from build123d import *

# Parameters (mm, degrees)
SKETCH1_R           = 14.3002
BOSS_EXTRUDE1_DEPTH = 69.85
SKETCH2_W           = 25.4
SKETCH2_H           = 44.45
CUT_EXTRUDE1_DEPTH  = 44.45
FILLET1_R           = 3.175
SKETCH3_R           = 2.921
CUT_EXTRUDE2_DEPTH  = 107.823534499
SKETCH4_R           = 2.921
CUT_EXTRUDE3_DEPTH  = 107.823534499
SKETCH5_R           = 4.445
CUT_EXTRUDE4_DEPTH  = 6.35
CUT_EXTRUDE5_DEPTH  = 7.62


with BuildPart() as part:
    # Sketch1 → Boss-Extrude1 (new body)
    with BuildSketch(Plane(origin=(0, 0, 0), x_dir=(0, 0, -1), z_dir=(1, 0, 0))):
        with BuildLine():
            Line((0, 0), (57.15, 0))
            Line((57.15, 0), (57.15, 38.1))
            ThreePointArc((57.15, 38.1), (51.570384182, 51.570384182), (38.1, 57.15))
            Line((38.1, 57.15), (0, 57.15))
            Line((0, 57.15), (0, 0))
        make_face()
        with Locations((31.75, 31.75)):
            Circle(SKETCH1_R, mode=Mode.SUBTRACT)
    extrude(amount=BOSS_EXTRUDE1_DEPTH)

    # Sketch2 → Cut-Extrude1 (cut)
    with BuildSketch(Plane(origin=(0, 57.15, 0), x_dir=(1, 0, 0), z_dir=(0, 1, 0))):
        with Locations((12.7, 34.925)):
            Rectangle(SKETCH2_W, SKETCH2_H)
        with Locations((57.15, 34.925)):
            Rectangle(SKETCH2_W, SKETCH2_H)
    extrude(amount=-CUT_EXTRUDE1_DEPTH, mode=Mode.SUBTRACT)

    # Fillet1
    fillet1_edges = [part.edges().sort_by_distance(p)[0] for p in [
        (69.85, 6.35, -57.15),
        (0, 57.15, -6.35),
        (69.85, 57.15, -6.35),
        (0, 12.7, -34.925),
        (0, 34.925, -12.7),
        (25.4, 25.4, -57.15),
        (25.4, 51.570384182, -51.570384182),
        (25.4, 12.7, -34.925),
        (12.7, 12.7, -57.15),
        (12.7, 12.7, -12.7),
        (25.4, 34.925, -12.7),
        (25.4, 57.15, -25.4),
        (12.7, 57.15, -12.7),
        (44.45, 51.570384182, -51.570384182),
        (44.45, 12.7, -34.925),
        (44.45, 34.925, -12.7),
        (69.85, 12.7, -34.925),
        (57.15, 12.7, -12.7),
        (69.85, 34.925, -12.7),
        (57.15, 12.7, -57.15),
        (44.45, 25.4, -57.15),
        (44.45, 57.15, -25.4),
        (57.15, 57.15, -12.7),
        (0, 6.35, -57.15),
        (34.925, 57.15, 0),
    ]]
    fillet(fillet1_edges, radius=FILLET1_R)

    # Sketch3 → Cut-Extrude2 (cut, through all)
    with BuildSketch(Plane.XY):
        with Locations((9.525, 25.4)):
            Circle(SKETCH3_R)
        with Locations((60.325, 25.4)):
            Circle(SKETCH3_R)
    extrude(amount=-CUT_EXTRUDE2_DEPTH, mode=Mode.SUBTRACT)

    # Sketch4 → Cut-Extrude3 (cut, through all)
    with BuildSketch(Plane.XZ):
        with Locations(Location((57.15, -25.4, 0), (0, 0, 270))):
            Circle(SKETCH4_R)
        with Locations(Location((57.15, -44.45, 0), (0, 0, 270))):
            Circle(SKETCH4_R)
        with Locations(Location((12.7, -25.4, 0), (0, 0, 270))):
            Circle(SKETCH4_R)
        with Locations(Location((12.7, -44.45, 0), (0, 0, 270))):
            Circle(SKETCH4_R)
    extrude(amount=-CUT_EXTRUDE3_DEPTH, mode=Mode.SUBTRACT)

    # Sketch5 → Cut-Extrude4 (cut)
    with BuildSketch(Plane(origin=(0, 12.7, 0), x_dir=(1, 0, 0), z_dir=(0, 1, 0))):
        with Locations(Location((12.7, 25.4, 0), (0, 0, 270))):
            Circle(SKETCH5_R)
        with Locations(Location((12.7, 44.45, 0), (0, 0, 270))):
            Circle(SKETCH5_R)
        with Locations(Location((57.15, 44.45, 0), (0, 0, 270))):
            Circle(SKETCH5_R)
        with Locations(Location((57.15, 25.4, 0), (0, 0, 270))):
            Circle(SKETCH5_R)
    extrude(amount=-CUT_EXTRUDE4_DEPTH, mode=Mode.SUBTRACT)

    # Sketch6 → Cut-Extrude5 (cut)
    with BuildSketch(Plane(origin=(0, 0, -12.7), x_dir=(-1, 0, 0), z_dir=(0, 0, -1))):
        Polygon((-57.392060633, 30.48), (-63.257939367, 30.48), (-66.190878735, 25.4), (-63.257939367, 20.32), (-57.392060633, 20.32), (-54.459121265, 25.4), align=None)
        Polygon((-6.592060633, 30.48), (-12.457939367, 30.48), (-15.390878735, 25.4), (-12.457939367, 20.32), (-6.592060633, 20.32), (-3.659121265, 25.4), align=None)
    extrude(amount=-CUT_EXTRUDE5_DEPTH, mode=Mode.SUBTRACT)


solid = part.part
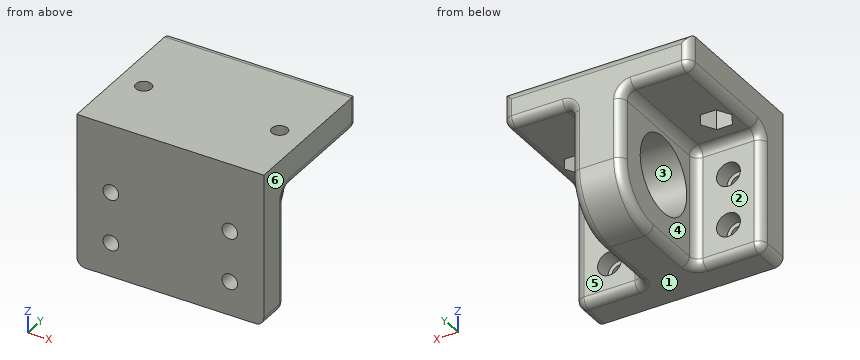
The listing builds one solid part. Answer for the finished solid, in the listing's coordinates (mm). Face numbers are marked on the shaded views. A direction names the side the tool comes from. Coordinates: 2 decimals unless noted, no trailing zeros. Write each loop counter-clockwise with the first axis right and the second up, starting at its lowest first coordinate (ties: lowest second). Pieces come first, ordered by that corner, then holes. Notation, with made-up numbers: M 46.5,36 L 99.5,36 A20 ccw 99.5,40 Z; hole C -24.75,6.25 d9. An arc over 180 degrees is marked long. Put each result on its own line as item: value. Start each with the question number.
1. A cutting plane is placed at C-C on z = -25. Count the separate pieces of the cut face and the enclosed holes in it, then the cut area to 3 significant figures.
2. Which of the six approach directions +Z, -Z, +X, -X, +Y, -Y give full straight-line access (tool end or side, diameter ignored) to the marked faces 4, 5 and 6?
3. For a pull along Z with two mould halves and no side action, classify the marked faces 1, 2 and 3 as pulls with the +Z half, pulls with the -Z half, needs draft (parallel to the pull), parting line crosses it, or undercut.
4. Consider line 1 (X direction, y = 3, z = -25.4); line 2 (Z direction, x = 57, y = 10); line 3 (X direction, y = 10.5, z = -23). Determine where each line is inside the solid, lowest interval first. Write a range as from..to.
5. Flat-ended cylindrical pins translate along their axes: P1, Ø23, axis at y = 31.75, z = -31.75, coming from the +X side (3 decimals); P2, Ø10, axis at y = 51.5, z = -43, coming from the +X side; P3, Ø10, axis at x = 46, y = 48, coming from the -Z side; P4, Ø1.5, axis at x = 12, y = 25.5, coming from the +Z side. Find the tip coordinate at first contact, or state that the pin passes through.
6. A cutting plane is placed at A-A on z = -31.75. Write down the section's boundary in (x, y) (3 decimals).
7. A cutting plane is placed at B-B on x = 38.5. Write down the section's boundary in (y, z) (3 decimals), then the cut area to 3 significant figures.
Resolved:
1. separate pieces: 4
1. enclosed holes: 0
1. area: 1,060 mm2
2. face 4: -Z, -X, +Y
2. face 5: -Z, +X, +Y
2. face 6: +Z, -Z, +X, +Y, -Y
3. face 1: pulls with the -Z half
3. face 2: needs draft
3. face 3: undercut
4. line 1: x = 0..9.78, 15.62..54.23, 60.07..69.85
4. line 2: z = -57.11..-48.89, -40.01..-29.84, -20.96..0
4. line 3: x = 0.15..8.96, 16.44..53.41, 60.89..69.7
5. P1: passes through
5. P2: stops at x = 44.45
5. P3: stops at z = -55.81
5. P4: stops at z = 0
6. outline: M 0,0 L 69.85,0 L 69.85,9.525 A3.175 ccw 66.675,12.7 L 47.625,12.7 A3.175 cw 44.45,15.875 L 44.45,17.45 L 25.4,17.45 L 25.4,15.875 A3.175 cw 22.225,12.7 L 3.175,12.7 A3.175 ccw 0,9.525 Z; M 25.4,46.05 L 44.45,46.05 L 44.45,53.975 A3.175 ccw 41.275,57.15 L 28.575,57.15 A3.175 ccw 25.4,53.975 Z
7. outline: M 0,-57.15 L 38.1,-57.15 A19.05 ccw 57.15,-38.1 L 57.15,-3.175 A3.175 ccw 53.975,0 L 0,0 Z; hole C 31.75,-31.75 d28.6
7. area: 2,540 mm2
